Read the model definition and answer for the solid it produces. Units are mm, in the model's axes. A direction names the side the tool comes from. Coordinates: 2 decimals unless noted, no trailing zeros. Write each loop counter-clockwise with the first axis right and the second up, starting at its lowest first coordinate (ties: lowest second). Pieces come first, ordered by that corner, then holes. Notation, with made-up numbers: (-27.5, 35.5) -> (-18.5, 35.5) arc R7 ccw to (-18.5, 42.5) -> close; hole circle Ø3 at (-9, 82.25). An arc over 180 degrees is marked (long way). Write item = value, one per line. Start each with the question number.
1) Section A-A (y = -9.25) is taken. Determine the outline of the cut face in (x, z), plus the area to 3 significant figures.
2) Find the intervals of material crossed by line 1 along Z through (x, y) = (-0.1, 2.5); line 2 along X through (y, z) = (4.75, 0.75); line 3 along X through (y, z) = (3, 1.55), in increasing order. Write a range as from..to.
3) A tool of negligible diameter and unlimited length cuts with its end or side. For faces 1 (the face through (-1, -12, 0)), 2 (the face through (-0.512, -5.916, -0.108)), from which of +Z, -Z, +X, -X, +Y, -Y can it reach the whole face along a straight path? Write none if from no direction.
4) Section B-B (y = 1.5) is taken. Determine the outline of the cut face in (x, z).
5) For a pull along X with two mould halves and no side action, classify faces 3 (the face through (1.3, -5.9, -0.4)), 4 (the face through (-2.44, 3.94, -0.54)), 5 (the face through (1, -12, 0)) as released by +X, released by -X, zero draft, split by the parting line, or undercut.
6) A flat-ended cylindrical pin translates along its axis: pin 1 Ø1.5 at (x, z) = (-1.5, 1.5) entering from -Y. Find the tip coordinate at first contact, or state that the pin passes through.
from build123d import *

# Parameters (mm, degrees)
SKETCH1_R           = 2.5
BOSS_EXTRUDE1_DEPTH = 8
SKETCH3_R           = 0.5
BOSS_EXTRUDE2_DEPTH = 12


with BuildPart() as part:
    # Sketch1 → Boss-Extrude1 (new body)
    with BuildSketch(Plane(origin=(0, 0, 0), x_dir=(1, 0, 0), z_dir=(0, 1, 0))):
        with Locations(Location((0, 0, 0), (0, 0, 270))):
            Circle(SKETCH1_R)
    extrude(amount=BOSS_EXTRUDE1_DEPTH)

    # Sketch2 → Cut-Revolve2 (revolve, cut)
    with BuildSketch(Plane.XY):
        Polygon((0, 8), (0, 6.5), (-2.5, 8), align=None)
    revolve(axis=Axis((0, 8, 0), (0, -1, 0)), mode=Mode.SUBTRACT)

    # Sketch3 → Boss-Extrude2 (add)
    with BuildSketch(Plane.XZ):
        with Locations(Location((-1, 0, 0), (0, 0, 90))):
            Circle(SKETCH3_R)
        with Locations(Location((1, 0, 0), (0, 0, 90))):
            Circle(SKETCH3_R)
    extrude(amount=BOSS_EXTRUDE2_DEPTH)


solid = part.part
Answer key:
q1.outline = circle Ø1 at (-1, 0); circle Ø1 at (1, 0)
q1.area = 1.57 mm^2
q2.line_1 = -2.5..2.5
q2.line_2 = -2.38..2.38
q2.line_3 = -1.96..1.96
q3.face_1 = +Z, -Z, +X, -X, -Y
q3.face_2 = -Y
q4.outline = circle Ø5 at (0, 0)
q5.face_3 = undercut
q5.face_4 = split by the parting line
q5.face_5 = zero draft
q6.pin_1 = 0
